Check sheet for the modelled part. Datum: model origin and axes. Units: mm. A direction names the side the tool comes from. Coordinates: 2 decimals unless noted, no trailing zeros. Write each loop counter-clockwise with the first axis right and the second up, starting at its lowest first coordinate (ties: lowest second). Pieces come first, ordered by that corner, then holes. Notation, with made-up numbers: (0.25, 72) -> (11.25, 72) arc R4 cw to (11.25, 77) -> close; hole circle Ø9 at (10, 23). An arc over 180 degrees is marked (long way). One line per item, written item: value. Start each with the question number.
1) Gauge pin test, flat ends, axial feed: P1, Ø12, axis at x = 12, z = -49, coming from the -Y side; P2, Ø10, axis at x = 4.5, z = -54.5, coming from the -Y side; P3, Ø6, axis at x = -10.5, z = 3, coming from the +Y side. Record the tip position at first contact, or that the pin passes through.
2) Sectioned sample at B-B on x = 20.5. Enter the section's corners in (y, z).
3) Sectioned sample at A-A on z = -105. Enter the section's corners in (x, y).
4) Set-up check for faces 1 (the flat face through (21, -15, -93)), 2 (the flat face through (21, 15, -93)), 3 (the flat face through (19, 28, -13)): record each of +Z, -Z, +X, -X, +Y, -Y from which the full face is reachable in a straight line by a thin tool's end or side.
5) Scan lines: line 1 along Z through (x, y) = (-8.5, 4); line 2 along X through (y, z) = (45, 25); line 3 along Y through (x, z) = (20, -84). Record each from-to range of solid material in increasing order. Write a range as [from, to].
```python
from build123d import *

# Parameters (mm, degrees)
BOSS_EXTRUDE1_DEPTH      = 19
BOSS_EXTRUDE1_DEPTH_BACK = 19
SKETCH4_R                = 25
BOSS_EXTRUDE2_DEPTH      = 4
SKETCH7_W                = 96.334868302
SKETCH7_H                = 30
BOSS_EXTRUDE4_DEPTH      = 4


with BuildPart() as part:
    # Sketch3 → Boss-Extrude1 (new body, two sides)
    with BuildSketch(Plane(origin=(0, 0, 0), x_dir=(0, 0, -1), z_dir=(1, 0, 0))) as boss_extrude1_sk:
        with BuildLine():
            Line((101.125836247, 15), (115.903665145, 15))
            Line((115.903665145, 15), (115.903665145, -15))
            Line((115.903665145, -15), (101.125836247, -15))
            add(Edge.make_bspline(
                [(-35.228525995, -21.228719453), (-33.006450865, -24.07111779), (-26.49753273, -26.863412426), (-11.335277797, -30.129234604), (12.719064979, -27.929719806), (43.096683762, -25.057564772), (73.387051738, -18.43106409), (92.126866656, -14.867150153), (101.125836247, -15)],
                knots=[0, 0, 0, 0, 0.075207413, 0.148741353, 0.333288022, 0.588928464, 0.80810625, 1, 1, 1, 1], degree=3))
            add(Edge.make_bspline(
                [(-30.278821492, 49.042821653), (-37.712518178, 26.883259009), (-45.501408919, 1.573924427), (-35.228525995, -21.228719453)],
                knots=[0, 0, 0, 0, 1, 1, 1, 1], degree=3))
            add(Edge.make_bspline(
                [(-30.278821492, 49.042821653), (-14.032986644, 49.168084942), (9.286633448, 46.599377579), (40.599784556, 39.089257371), (60.084206577, 29.540337779), (80.216148289, 20.129950878), (93.055643568, 15.237102325), (101.125836247, 15)],
                knots=[0, 0, 0, 0, 0.354356982, 0.512751412, 0.701525574, 0.826928454, 1, 1, 1, 1], degree=3))
        make_face()
    extrude(amount=BOSS_EXTRUDE1_DEPTH)
    extrude(boss_extrude1_sk.sketch, amount=-BOSS_EXTRUDE1_DEPTH_BACK)

    # Sketch4 → Boss-Extrude2 (add)
    with BuildSketch(Plane(origin=(19, 0, 0), x_dir=(0, 0, -1), z_dir=(1, 0, 0))):
        Circle(SKETCH4_R)
    extrude(amount=BOSS_EXTRUDE2_DEPTH)

    # Sketch7 → Boss-Extrude4 (add)
    with BuildSketch(Plane(origin=(19, 0, 0), x_dir=(0, 0, -1), z_dir=(1, 0, 0))):
        with Locations((67.736230994, 0)):
            Rectangle(SKETCH7_W, SKETCH7_H)
    extrude(amount=BOSS_EXTRUDE4_DEPTH)


solid = part.part
```
Answers:
1. P1: stops at y = -24.4
1. P2: stops at y = -23.31
1. P3: stops at y = 47.87
2. outline: (-15, -115.9) -> (15, -115.9) -> (15, -20) arc R25 ccw (long way) to (-15, -20) -> close
3. outline: (-19, -15) -> (23, -15) -> (23, 15) -> (-19, 15) -> close
4. face 1: -Z, +X, -Y
4. face 2: -Z, +X, +Y
4. face 3: +X
5. line 1: z = [-115.9, 40.16]
5. line 2: x = [-19, 19]
5. line 3: y = [-15, 15]
